Answer from the drawing. Dimensions are ordinates in mm from the lowest x, y and z of the part. A direction names the side the tool comes from. Coordinates: 2 decimals unless noted, no trailing zeros. Order: outer loops, then holes, each group sorted by start corner. A loop starts at its lowest first (then second) coordinate and runs counter-clockwise, first axis right, second up. Notation, with made-up numbers: (-3.5, -29) - (16.5, -29) arc R32 ccw to (16.5, 5) - close; hole circle Ø7 at (20.5, -32). An arc over 180 degrees is marked (long way). Answer as a JSON object with one key per item and string values. Group by question number.
1) The mould has two halves that part along X. Classify the marked faces 1, 2 and 3: released by +X, released by -X, zero draft, split by the parting line, or undercut.
2) Section A-A (z = 4) is taken. Give the vertices of the cut face in (x, y).
3) Find the intervals of material crossed by line 1 along X through (y, z) = (2.75, 4); line 2 along X through (y, z) = (1.4, 4); line 3 along Z through (x, y) = (3, 5.3), in increasing order.
4) A tool of negligible diameter and unlimited length cuts with its end or side. For the marked faces 4 and 5, from which of +Z, -Z, +X, -X, +Y, -Y can it reach the whole face along a straight path? Write none if from no direction.
5) Section D-D (y = 4) is taken. Give the vertices of the cut face in (x, z), plus the area to 3 significant figures.
6) Section C-C (y = 0.5) is taken. Give the vertices of the cut face in (x, z).
7) This flat-tipped pin is pushed along its axis until it touches: P1, Ø2, axis at y = 1.5, z = 6.5, coming from the -X side. Where does it stop, or does it pass through?
8) Section B-B (x = 4) is taken. Give the vertices of the cut face in (y, z).
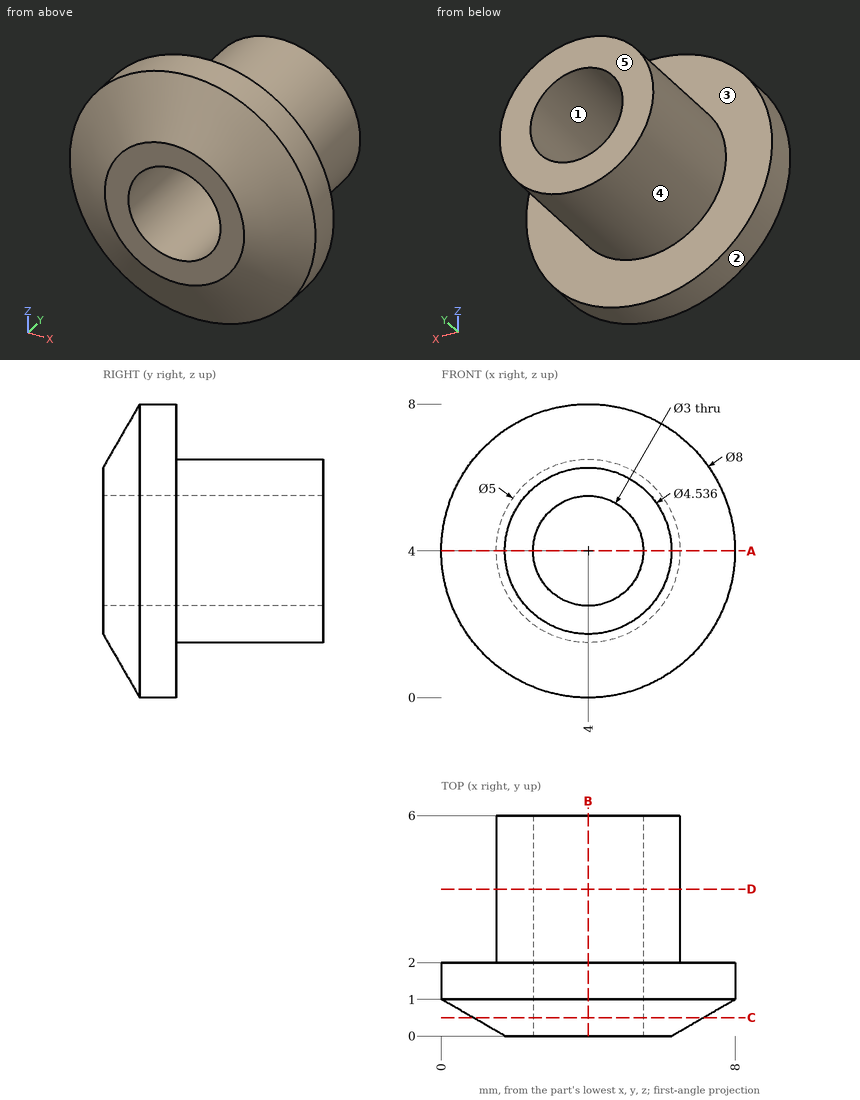
Report:
{
 "1": {"face 1": "undercut", "face 2": "split by the parting line", "face 3": "zero draft"},
 "2": {"outline": "(0, 1) - (1.73, 0) - (2.5, 0) - (2.5, 6) - (1.5, 6) - (1.5, 2) - (0, 2) - close; (5.5, 0) - (6.27, 0) - (8, 1) - (8, 2) - (6.5, 2) - (6.5, 6) - (5.5, 6) - close"},
 "3": {"line 1": "x = 1.5 to 2.5, 5.5 to 6.5", "line 2": "x = 0 to 2.5, 5.5 to 8", "line 3": "z = 1.71 to 2.88, 5.12 to 6.29"},
 "4": {"face 4": "+Y", "face 5": "+Z, -Z, +X, -X, +Y"},
 "5": {"outline": "circle Ø5 at (4, 4); hole circle Ø3 at (4, 4)", "area": "12.6 mm²"},
 "6": {"outline": "circle Ø6.27 at (4, 4); hole circle Ø3 at (4, 4)"},
 "7": {"P1": "stops at x = 0.29"},
 "8": {"outline": "(0, 1.73) - (1, 0) - (2, 0) - (2, 1.5) - (6, 1.5) - (6, 2.5) - (0, 2.5) - close; (0, 5.5) - (6, 5.5) - (6, 6.5) - (2, 6.5) - (2, 8) - (1, 8) - (0, 6.27) - close"}
}
